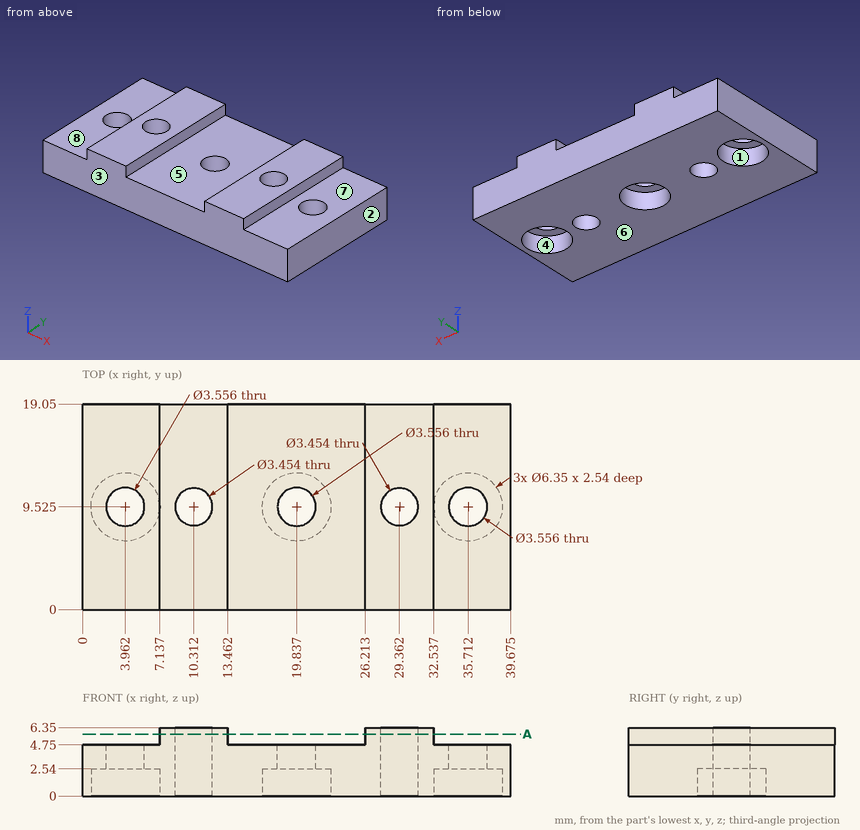
Here's the drawing with two shaded views (mm, measured from the low corner). I have some questions. A direction names the side the tool comes from. Round coordinates to 2 decimals unless told otherwise and drop trailing zeros.
Item 1: Please list where these lines run through material, in increasing order: L1, parallel to X at y = 12.75, z = 5.5; L2, parallel to X at y = 9.5, z = 2.25 (1 decimal); L3, parallel to Y at x = 11, z = 3.25.
Item 2: Which directions (+Z, -Z, +X, -X, +Y, -Y) give clear straight access to the entire face, cutting with the end or side of a thin tool? Please do the marked faces 4, 5, 6, 7 and 8.
Item 3: If we mould it in two halves opening along Y, with no side actions, what happens to the marked faces 1, 2 and 3? For each: +Y half, -Y half, draft (parallel to the pull), parting line (faces both ways), or undercut.
Item 4: Suppose I cut it at A-A, the plane z = 5.75. State how many separate pieces and enclosed holes the cut face has, then the cut area to 3 significant figures.
Item 5: Will these pins go through, and if not, where does the flat tip stop? pin 1 Ø5 at (x, y) = (3.96, 9.52) entering from +Z; pin 2 Ø5.5 at (x, y) = (19.84, 9.52) entering from -Z; pin 3 Ø0.8 at (y, z) = (6, 6) entering from +X.
Reported:
1. L1: x = 7.14 to 13.46, 26.21 to 32.54
1. L2: x = 0 to 0.8, 7.1 to 8.6, 12 to 16.7, 23 to 27.6, 31.1 to 32.5, 38.9 to 39.7
1. L3: y = 0 to 7.94, 11.11 to 19.05
2. face 4: -Z
2. face 5: +Z, +Y, -Y
2. face 6: -Z, +X, -X, +Y, -Y
2. face 7: +Z, +X, +Y, -Y
2. face 8: +Z, -X, +Y, -Y
3. face 1: undercut
3. face 2: draft
3. face 3: -Y half
4. separate pieces: 2
4. enclosed holes: 2
4. area: 222 mm2
5. pin 1: stops at z = 4.75
5. pin 2: stops at z = 2.54
5. pin 3: stops at x = 32.54
